Read the model definition and answer for the solid it produces. Units are mm, in the model's axes. A direction names the side the tool comes from. Give positions to 0.01 mm unless a question says otherwise; leave off trailing zeros. Order: outer loops, then holes, each group sorted by start corner. A loop starts at its lowest first (then second) coordinate and runs counter-clockwise, first axis right, second up. Notation, with made-up numbers: (41.25, 47.5) -> (56.25, 47.5) arc R13 cw to (56.25, 65.5) -> close; hole circle Ø6 at (65.25, -40). An arc over 180 degrees is marked (long way). Use one line per item in the form item = value.
Autodesk Inventor part; units mm, degrees
ref_plane "WorkPlane1" through (0, 0, 0) normal (0, 0, 1) x (1, 0, 0)
ref_plane "Work Plane2" through (0, 0, -2) normal (0, 0, 1) x (1, 0, 0)
ref_plane "WorkPlane2" through (0, 0, 1) normal (0, 0, 1) x (1, 0, 0)
ref_plane "WorkPlane1" through (0, 0, 0) normal (0, 0, 1) x (1, 0, 0)
ref_plane "Work Plane2" through (0, 0, -2) normal (0, 0, 1) x (1, 0, 0)
ref_plane "WorkPlane2" through (0, 0, 1) normal (0, 0, 1) x (1, 0, 0)
sketch "Sketch1" plane through (0, 0, 0) normal (0, 0, 1) x (1, 0, 0)
  point P0 (0, 0)
sketch "Sketch2" plane through (0, 0, 0) normal (0, 0, 1) x (1, 0, 0)
  line L0 (6.5, -25.6418) -> (5.6643, -22.1866)
  arc A0 (9.3096, -19.9443) -> (5.6643, -22.1866) centre (7.8513, -21.6577) ccw
  line L1 (9.3096, -19.9443) -> (11.7235, -21.9989)
  arc A1 (11.7235, -21.9989) -> (-11.7235, -21.9989) centre (0, 0) ccw
  line L2 (-9.3096, -19.9443) -> (-11.7235, -21.9989)
  arc A2 (-5.6643, -22.1866) -> (-9.3096, -19.9443) centre (-7.8513, -21.6577) ccw
  line L3 (-6.5, -25.6418) -> (-5.6643, -22.1866)
  arc A3 (6.5, -25.6418) -> (-6.5, -25.6418) centre (0, 1.2333) ccw
  line L4 (0, 1.2333) -> (-6.5, -25.6418) construction
  line L5 (0, 1.2333) -> (6.5, -25.6418) construction
  dimension "d2" = 27.65
  dimension "d4" = 0
  dimension "d6" = 24.9278
  dimension "d8" = 1.2333
  dimension "d10" = 6.5
  dimension "d12" = 6.5
  dimension "d14" = 2.25
  dimension "d16" = 2.25
  dimension "d18" = 24.2
  dimension "d20" = 24.2
  dimension "d22" = 36
  dimension "d24" = 36
extrude "Extrusion1" add sketch "Sketch2" along normal blind 2
sketch "Sketch3" plane through (0, 0, 2) normal (0, 0, 1) x (1, 0, 0)
  arc A0 (-5.6643, -22.1866) -> (-9.3096, -19.9443) centre (-7.8513, -21.6577) ccw
hole "Hole1" at (-7.8513, -21.6577, 2) direction (0, 0, -1) diameter 2.5 end through all
sketch "Sketch4" plane through (0, 0, 2) normal (0, 0, 1) x (1, 0, 0)
  arc A0 (9.3096, -19.9443) -> (5.6643, -22.1866) centre (7.8513, -21.6577) ccw
hole "Hole2" at (7.8513, -21.6577, 2) direction (0, 0, -1) diameter 2.5 end through all
equation "\"d29\" = Diam5"
equation "\"d36\" = Diam5"
equation "\"d2\" = 0.5 * Diam2"
equation "\"d6\" = 0.5 * msp_dd1"
equation "\"d8\" = -0.5 * msp_dd1 + 0.5 * Diam2 - 0.222222 * ParA"
equation "\"d10\" = 2.6 * Diam5"
equation "\"d12\" = 2.6 * Diam5"
equation "\"d14\" = 0.9 * Diam5"
equation "\"d16\" = 0.9 * Diam5"
equation "\"d18\" = 1.3 * Diam5 + 0.5 * Diam2 - ParA"
equation "\"d20\" = 1.3 * Diam5 + 0.5 * Diam2 - ParA"
equation "\"d25\" = ParS"
equation "\"Diam5\" = 2.5"
equation "\"ParA\" = 6.7"
equation "\"ParS\" = 2"
equation "\"Diam2\" = 55.3"
equation "\"msp_dd1\" = -b + Diam2 - 0.111111 * ParA"
equation "\"msp_pom\" = 0.5 * Diam2 - b"
equation "\"TEMPLATE\" = 1.2345"
properties part number "ANSI B 27.7M - 3BMI-52" material "Steel, Mild"
Item 1: The part is cut by section D-D on x = 0. Give the vertices of the cut face in (y, z), and give its area (3 significant figures).
Checks:
outline = (24.93, 0) -> (28.88, 0) -> (28.88, 2) -> (24.93, 2) -> close
area = 7.91 mm²
Item 2: Determine the mould class of faces 4 (the cylindrical face through (-1.12, 28.86, 0.99)), 5 (the flat face through (-10.5, -20.96, 0.99)), 6 (the flat face through (8, 24, 0)), 7 (the flat face through (-6.09, -23.94, 0.99)) for opening direction Y: +Y half, -Y half, draft (parallel to the pull), parting line (faces both ways), or undercut.
Checks:
face_4 = parting line
face_5 = undercut
face_6 = draft
face_7 = -Y half
Item 3: The part is cut by section A-A on x = -13. Give the vertices of the cut face in (y, z).
Checks:
outline = (-23.17, 0) -> (-21.27, 0) -> (-21.27, 2) -> (-23.17, 2) -> close; (21.27, 0) -> (25.64, 0) -> (25.64, 2) -> (21.27, 2) -> close
Item 4: The part is cut by section C-C on z = 0.95. Give the vertices of the cut face in (x, y).
Checks:
outline = (-11.72, -22) arc R24.93 cw (long way) to (11.72, -22) -> (9.31, -19.94) arc R2.25 ccw to (5.66, -22.19) -> (6.5, -25.64) arc R27.65 ccw (long way) to (-6.5, -25.64) -> (-5.66, -22.19) arc R2.25 ccw to (-9.31, -19.94) -> close; hole circle Ø2.5 at (-7.85, -21.66); hole circle Ø2.5 at (7.85, -21.66)
Item 5: Which of the six approach directions +Z, -Z, +X, -X, +Y, -Y give full straight-line access (tool end or side, diameter ignored) to faces 1 (the flat face through (10.5, -20.96, 0.99)), 2 (the flat face through (8, 24, 2)), 3 (the flat face through (6.09, -23.94, 0.99))?
Checks:
face_1 = +Z, -Z
face_2 = +Z, +X, -X, +Y, -Y
face_3 = +Z, -Z, -Y
Item 6: Given pin 1 Ø10 at (x, y) = (16, -18) entering from -Z, flat-ended and moving along its own axis, determine where the tip first touches the part or whether it passes through.
Checks:
pin_1 = 0
Item 7: Straight lines are drawn through the part: L1, parallel to Y at x = 8, z = 0.9; L2, parallel to Y at x = 15, z = 1.95; L3, parallel to Y at x = -11, z = 1.3. For each, find the intervals that lie inside material, in ascending order. Write a range as from..to.
Checks:
L1 = -25.23..-22.9, -20.42..-19.41, 23.61..27.7
L2 = -21.99..-19.91, 19.91..24.46
L3 = -24.13..-21.38, 22.37..26.6
Item 8: The part is cut by section B-B on y = -10.5. Give the vertices of the cut face in (x, z), and give its area (3 significant figures).
Checks:
outline = (-25.04, 0) -> (-22.61, 0) -> (-22.61, 2) -> (-25.04, 2) -> close; (22.61, 0) -> (25.04, 0) -> (25.04, 2) -> (22.61, 2) -> close
area = 9.71 mm²
